Study the drawing (mm; zero at the part's minimum x, y, z) and answer. Round coordinates to 2 decimals unless told otherwise and drop trailing zeros. Order: outer loops, then holes, each group sorted by start corner. A loop starts at its lowest first (then second) coordinate and runs counter-clockwise, first axis right, second up. Notation, with made-up numbers: (60.25, 41.25) -> (97.25, 41.25) arc R31 ccw to (97.25, 67.25) -> close; hole circle Ø3 at (0, 6.25). An arc over 180 degrees is marked (long way). Answer in a Markdown table with one row per item. Add a question column.
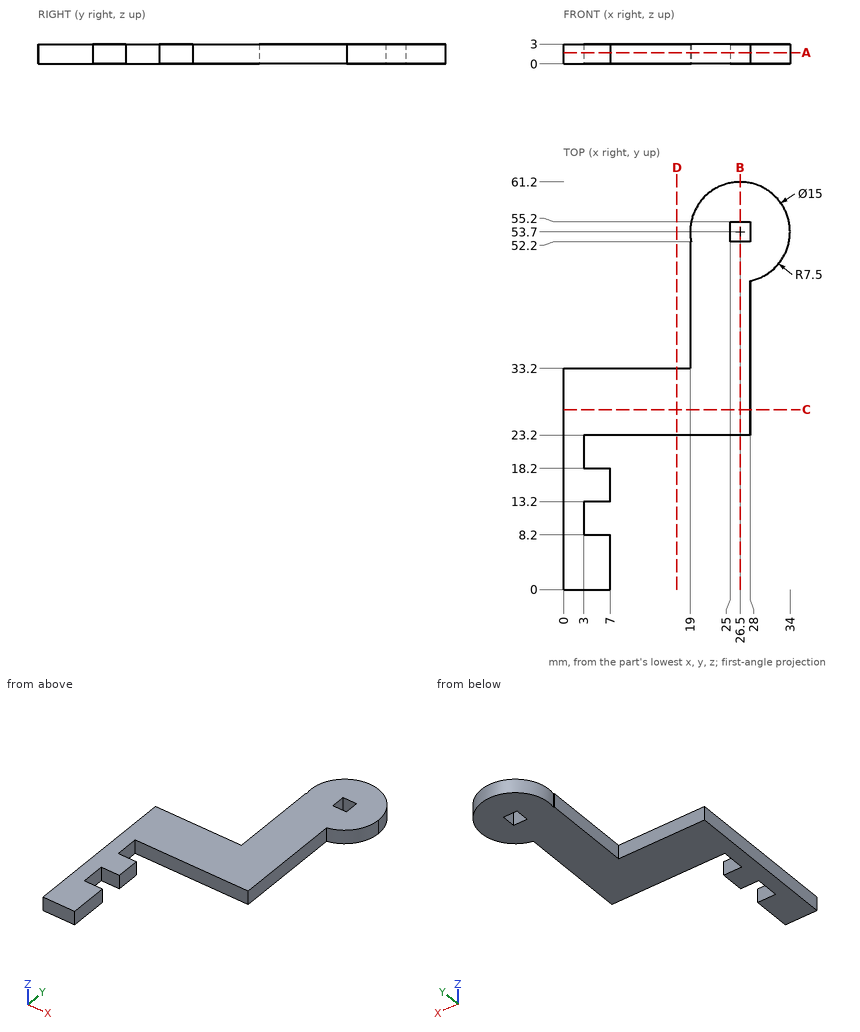
Item 1: The part is cut by section D-D, the plane x = 17. Give the vertices of the cut face in (y, z).
Item 2: The part is cut by section C-C, the plane y = 27. Give the vertices of the cut face in (x, z), and give its area (3 significant figures).
Item 3: Find the intervals of material crossed by probe 1 along Y at (x, z) = (26.5, 2); probe 2 along X at (y, z) = (5, 1.6); probe 3 along X at (y, z) = (12.5, 2.8), in increasing order. Write a range as [from, to].
Item 4: Flat-ended cylindrical pins translate along their axes: P1, Ø1.5, axis at y = 10.5, z = 2, coming from the +X side; P2, Ø0.9, axis at y = 16.5, z = 2, coming from the +X side; P3, Ø1.5, axis at y = 43, z = 0.5, coming from the +X side. Find the tip coordinate at first contact, or state that the pin passes through.
Item 5: The part is cut by section A-A, the plane z = 1.7. Give the vertices of the cut face in (x, y), and give its area (3 significant figures).
Item 6: The part is cut by section B-B, the plane x = 26.5. Give the vertices of the cut face in (y, z).
Resolved:
| question | item | result |
|---|---|---|
| 1 | outline | (23.2, 0) -> (33.2, 0) -> (33.2, 3) -> (23.2, 3) -> close |
| 2 | outline | (0, 0) -> (28, 0) -> (28, 3) -> (0, 3) -> close |
| 2 | area | 84.0 mm2 |
| 3 | probe 1 | [23.2, 52.2], [55.2, 61.2] |
| 3 | probe 2 | [0, 7] |
| 3 | probe 3 | [0, 3] |
| 4 | P1 | x = 3 |
| 4 | P2 | x = 7 |
| 4 | P3 | x = 28 |
| 5 | outline | (0, 0) -> (7, 0) -> (7, 8.2) -> (3, 8.2) -> (3, 13.2) -> (7, 13.2) -> (7, 18.2) -> (3, 18.2) -> (3, 23.2) -> (28, 23.2) -> (28, 46.35) arc R7.5 ccw (long way) to (19.15, 52.2) -> (19, 52.2) -> (19, 33.2) -> (0, 33.2) -> close; hole (25, 52.2) -> (28, 52.2) -> (28, 55.2) -> (25, 55.2) -> close |
| 5 | area | 699 mm2 |
| 6 | outline | (23.2, 0) -> (52.2, 0) -> (52.2, 3) -> (23.2, 3) -> close; (55.2, 0) -> (61.2, 0) -> (61.2, 3) -> (55.2, 3) -> close |
